from build123d import *

# Parameters (mm, degrees)
RESSALTO_EXTRUS_O1_DEPTH = 327.5
ESBO_O2_R                = 8
CORTE_EXTRUS_O1_DEPTH    = 655
RESSALTO_EXTRUS_O2_DEPTH = 25
RESSALTO_EXTRUS_O3_DEPTH = 25
CHANFRO1_SIZE            = 50
CHANFRO1_SIZE2           = 8.816349035
CORTE_EXTRUS_O2_START    = -48
CORTE_EXTRUS_O2_DEPTH    = 48
CHANFRO2_SIZE            = 3


with BuildPart() as part:
    # Esboço1 → Ressalto-extrusão1 (new, symmetric)
    with BuildSketch(Plane.XY):
        Polygon((-19, 0), (19, 0), (19, 6), (24, 6), (24, -30), (-24, -30), (-24, 6), (-19, 6), align=None)
    extrude(amount=RESSALTO_EXTRUS_O1_DEPTH, both=True)

    # Esboço2 → Corte-extrusão1 (cut)
    with BuildSketch(Plane(origin=(24, 0, 0), x_dir=(0, 0, -1), z_dir=(1, 0, 0))):
        with Locations(Location((-297.5, -15, 0), (0, 0, 90))):
            Circle(ESBO_O2_R)
        with Locations(Location((297.5, -15, 0), (0, 0, 90))):
            Circle(ESBO_O2_R)
        with Locations(Location((-1.5, -15, 0), (0, 0, 90))):
            Circle(ESBO_O2_R)
    extrude(amount=-CORTE_EXTRUS_O1_DEPTH, mode=Mode.SUBTRACT)

    # Esboço3 → Ressalto-extrusão2 (add)
    with BuildSketch(Plane.XY.offset(327.5)):
        Polygon((-24, 6), (-24, -30), (24, -30), (24, 6), (19, 6), (19, 0), (-19, 0), (-19, 6), align=None)
    extrude(amount=RESSALTO_EXTRUS_O2_DEPTH)

    # Esboço4 → Ressalto-extrusão3 (add)
    with BuildSketch(Plane(origin=(0, 0, -327.5), x_dir=(-1, 0, 0), z_dir=(0, 0, -1))):
        Polygon((24, -30), (24, 6), (19, 6), (19, 0), (-19, 0), (-19, 6), (-24, 6), (-24, -30), align=None)
    extrude(amount=RESSALTO_EXTRUS_O3_DEPTH)

    # Chanfro1
    chanfro1_edges = [part.edges().sort_by_distance(p)[0] for p in [
        (0, 0, 352.5),
        (0, 0, -352.5),
    ]]
    chanfro1_side = [part.faces().sort_by_distance(p)[0] for p in [
        (0, 0, 0),
    ]]
    chamfer(chanfro1_edges, length=CHANFRO1_SIZE, length2=CHANFRO1_SIZE2, reference=chanfro1_side[0])

    # Esboço5 → Corte-extrusão2 (cut)
    with BuildSketch(Plane(origin=(24, 0, 0), x_dir=(0, 0, -1), z_dir=(1, 0, 0)).offset(CORTE_EXTRUS_O2_START)):
        Polygon((-352.5, -2.723789364), (-303.024931981, 6), (-352.5, 6), align=None)
        Polygon((352.5, 6), (352.5, -2.723789364), (303.024931981, 6), align=None)
    extrude(amount=CORTE_EXTRUS_O2_DEPTH, mode=Mode.SUBTRACT)

    # Chanfro2
    chanfro2_edges = [part.edges().sort_by_distance(p)[0] for p in [
        (24, -30, 0),
        (-24, -30, 0),
    ]]
    chamfer(chanfro2_edges, length=CHANFRO2_SIZE)


solid = part.part
CAD build for the part. Positions are in the model's coordinates, mm. A direction names the side the tool comes from. Coordinates: 2 decimals unless noted, no trailing zeros. Loops run counter-clockwise (first coordinate to the right, second up) from the corner with the lowest first, then second, coordinate; pieces in that order, holes last. Notation, with made-up numbers: (-14.75, 15) - (12.25, 15) arc R32 cw to (12.25, 47) - close; hole circle Ø1 at (88.25, 85.25). An arc over 180 degrees is marked (long way). Write item = value, one per line. Start each with the question number.
Q1. Cut at A-A, the plane y = -15. List the corners of the cut face in (x, z).
Q2. Pull direction Y, two halves, no side cores. Call faces 6 (the cylindrical face through (0.336, -16.041, -289.568)), 7 (the flat face through (-19, 2, 5)), 8 (the flat face through (0, -30, 5)): pulls with the +Y half, pulls with the -Y half, needs draft (parallel to the pull), parting line crosses it, or undercut.
Q3. Drill centre lines: L1, parallel to Z at x = -3, y = -15; L2, parallel to Y at x = 10, z = 1; L3, parallel to X at y = 2.5, z = 107. Where is each one in solid material? Low to high.
Q4. Flat gauge pin, fed straight in: pin 1 Ø8 at (x, z) = (-14, 264.5) entering from +Y. Where does the tip first touch, or does it go through?
Q5. Cut at C-C, the plane z = -114.5. List the corners of the cut face in (x, y), then the cut area to 3 significant figures.
Q6. Which spindle directions (+Z, -Z, +X, -X, +Y, -Y) get a long thin tool onto all of the face, cutting with end or side? Do faces 1 (the cylindrical face through (0.336, -16.041, 305.432)), 2 (the flat face through (0.27, -4.47, 327.85)), 3 (the flat face through (-0.27, -4.47, -327.85)), 4 (the flat face through (0, -19, -352.5)), 5 (the flat face through (0, 0, 4)). Say none if no direction does.
Q7. Cut at B-B, the plane x = -1.5. List the corners of the cut face in (y, z), then the cut area to 3 significant figures.
Computed:
q1.outline = (-24, -352.5) - (24, -352.5) - (24, -305.5) - (-24, -305.5) - close; (-24, -289.5) - (24, -289.5) - (24, -6.5) - (-24, -6.5) - close; (-24, 9.5) - (24, 9.5) - (24, 289.5) - (-24, 289.5) - close; (-24, 305.5) - (24, 305.5) - (24, 352.5) - (-24, 352.5) - close
q2.face_6 = undercut
q2.face_7 = needs draft
q2.face_8 = pulls with the -Y half
q3.L1 = -352.5 to -305.5, -289.5 to -6.5, 9.5 to 289.5, 305.5 to 352.5
q3.L2 = -30 to -22.98, -7.02 to 0
q3.L3 = -24 to -19, 19 to 24
q4.pin_1 = 0
q5.outline = (-24, -27) - (-21, -30) - (21, -30) - (24, -27) - (24, 6) - (19, 6) - (19, 0) - (-19, 0) - (-19, 6) - (-24, 6) - close
q5.area = 1,490 mm²
q6.face_1 = +X, -X
q6.face_2 = +Z, +Y
q6.face_3 = -Z, +Y
q6.face_4 = -Z, +X, -X, +Y, -Y
q6.face_5 = +Z, -Z, +Y
q7.outline = (-30, -352.5) - (-8.82, -352.5) - (0, -302.5) - (0, 302.5) - (-8.82, 352.5) - (-30, 352.5) - close; hole circle Ø16 at (-15, -297.5); hole circle Ø16 at (-15, 1.5); hole circle Ø16 at (-15, 297.5)
q7.area = 20,100 mm²
